Build history of the part. All positions in model axes, mm. Face numbers are marked on the shaded views. A direction names the side the tool comes from. Coordinates: 2 decimals unless noted, no trailing zeros. Write each loop counter-clockwise with the first axis right and the second up, starting at its lowest first coordinate (ties: lowest second). Pieces come first, ordered by that corner, then holes.
```python
from build123d import *

# Parameters (mm, degrees)
ESBO_O1_W                = 35
ESBO_O1_H                = 18
RESSALTO_EXTRUS_O1_DEPTH = 1.5
RESSALTO_EXTRUS_O2_DEPTH = 6.2
ESBO_O1_4_W              = 9
ESBO_O1_4_H              = 8
RESSALTO_EXTRUS_O3_DEPTH = 1.25


with BuildPart() as part:
    # Esbo_o1 → Ressalto-extrus_o1 (new body)
    with BuildSketch(Plane.XY):
        with Locations((17.5, 9)):
            Rectangle(ESBO_O1_W, ESBO_O1_H)
        Polygon((34, 1.477317564), (34, 9), (34, 17), (3, 17), (3, 1.477317564), align=None, mode=Mode.SUBTRACT)
    extrude(amount=RESSALTO_EXTRUS_O1_DEPTH)

    # Esbo_o1_3 → Ressalto-extrus_o2 (add)
    with BuildSketch(Plane.XY):
        Polygon((3, 1.477317564), (34, 1.477317564), (34, 9), (34, 17), (3, 17), align=None)
    extrude(amount=RESSALTO_EXTRUS_O2_DEPTH)

    # Esbo_o1_4 → Ressalto-extrus_o3 (add, symmetric)
    with BuildSketch(Plane.XY):
        with Locations((39.5, 7)):
            Rectangle(ESBO_O1_4_W, ESBO_O1_4_H)
    extrude(amount=RESSALTO_EXTRUS_O3_DEPTH, both=True)


solid = part.part
```
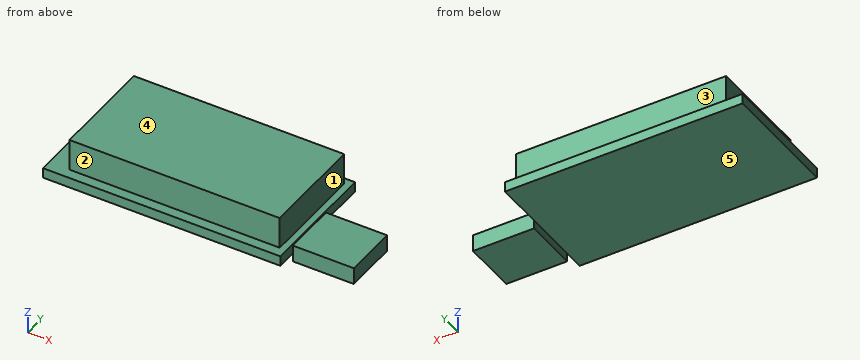
1. Saw through at A-A on y = 3.75. List the corners of the cut face in (x, z), plus the area to 3 significant figures.
Computed values:
outline: (0, 0) - (35, 0) - (35, -1.25) - (44, -1.25) - (44, 1.25) - (35, 1.25) - (35, 1.5) - (34, 1.5) - (34, 6.2) - (3, 6.2) - (3, 1.5) - (0, 1.5) - close
area: 221 mm2
2. Saw through at B-B on x = 9. List the corners of the cut face in (y, z).
Computed values:
outline: (0, 0) - (18, 0) - (18, 1.5) - (17, 1.5) - (17, 6.2) - (1.48, 6.2) - (1.48, 1.5) - (0, 1.5) - close
3. Flat gauge pins, fed straight in: pin 1 (2 mm diameter, centred on x = 40.5, z = 0.5, fed in from -Y); pin 2 (1.5 mm diameter, centred on x = 21.5, z = 4, fed in from -Y); pin 3 (3 mm diameter, centred on y = 15.5, z = 2, fed in from +X). Where does each tip first touch, or does it go through?
Computed values:
pin 1: stops at y = 3
pin 2: stops at y = 1.48
pin 3: stops at x = 35
4. Saw through at C-C on z = 5.75. List the corners of the cut face in (x, y).
Computed values:
outline: (3, 1.48) - (34, 1.48) - (34, 17) - (3, 17) - close
5. 3-axis set-ups, long thin cutter, end or side, ignore diameter. For the marked faces 1, 2, 3, 4 and 5: which of +Z, -Z, +X, -X, +Y, -Y reach the whole face in a straight line?
Computed values:
face 1: +Z, +X, +Y, -Y
face 2: +Z, +X, -X, -Y
face 3: +Z, +X, -X, +Y
face 4: +Z, +X, -X, +Y, -Y
face 5: -Z, -X, +Y, -Y
6. Probe line 1 along Z through (x, y) = (8, 1); line 2 along Y through (x, z) = (4, 4); line 3 along Z through (x, y) = (8.5, 12.5). List the from-to ranges inside material, lowest first.
Computed values:
line 1: z = 0 to 1.5
line 2: y = 1.48 to 17
line 3: z = 0 to 6.2
7. Saw through at D-D on y = 16.5. List the corners of the cut face in (x, z).
Computed values:
outline: (0, 0) - (35, 0) - (35, 1.5) - (34, 1.5) - (34, 6.2) - (3, 6.2) - (3, 1.5) - (0, 1.5) - close
